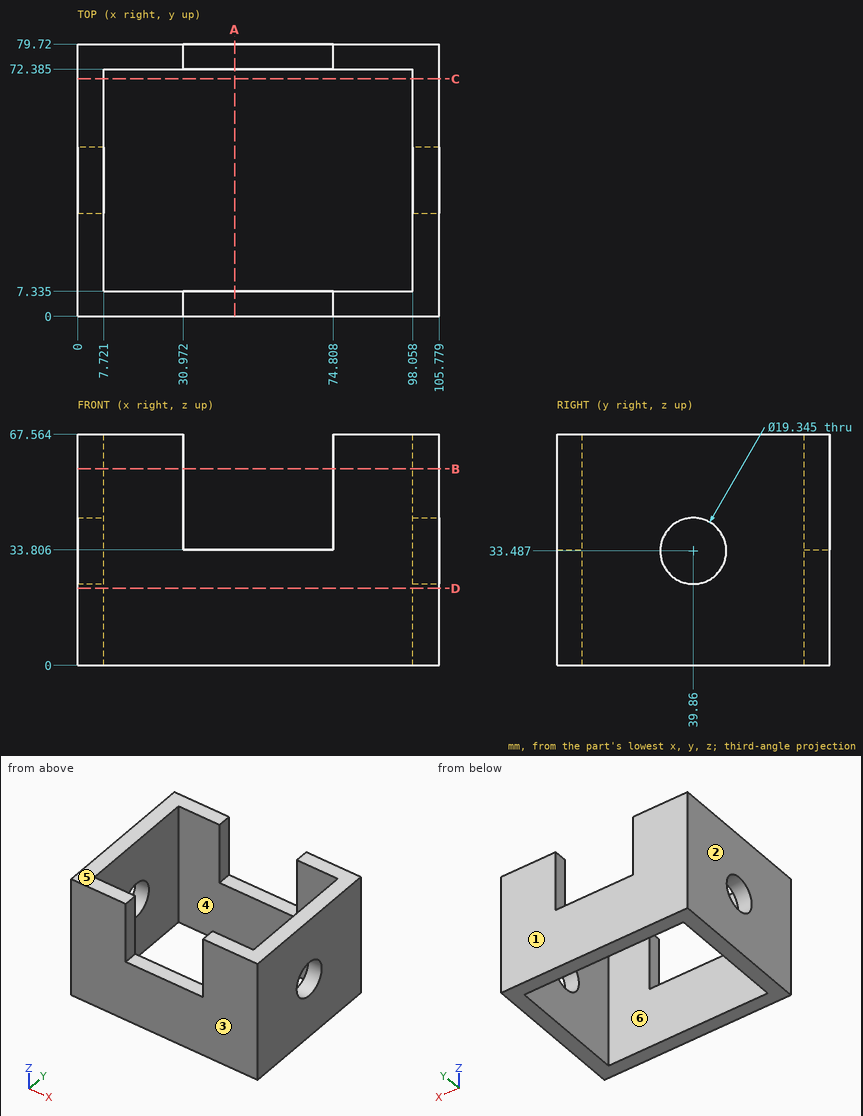
The figure shows three views and two pictorial views of one solid part (mm, origin at its lowest corner). Answer the questions. A direction names the side the tool comes from. Give positions to 0.01 mm unless a question says otherwise; leave off trailing zeros. Write each loop counter-clockwise with the first axis right and the second up, starting at its lowest first coordinate (ties: lowest second). Pieces come first, ordered by that corner, then holes. Notation, with made-up numbers: M -34.5,87.25 L 2.5,87.25 A15 cw 2.5,100.25 Z; hole C 23.5,62.5 d7. An arc over 180 degrees is marked long. One line per item, written item: value. Start each with the question number.
(1) A flat-ended cylindrical pin translates along its axis: pin 1 Ø6 at (x, y) = (47, 3.5) entering from +Z. Find the tip coordinate at first contact, or state that the pin passes through.
(2) Determine the mould class of the marked faces 1, 2, 3 and 4 for opening direction Y: pulls with the +Y half, pulls with the -Y half, needs draft (parallel to the pull), parting line crosses it, or undercut.
(3) Find the intervals of material crossed by line 1 (X direction, y = 30.5, z = 60.5); line 2 (Y direction, x = 94.5, z = 30) (1 decimal); line 3 (Z direction, x = 66.5, y = 73.5) (1 decimal), in increasing order.
(4) Find section B-B (z = 57.5). Determine the outline of the cut face in (x, y) (1 decimal).
(5) A tool of negligible diameter and unlimited length cuts with its end or side. For the marked faces 5 and 6, from which of +Z, -Z, +X, -X, +Y, -Y can it reach the whole face along a straight path? Write none if from no direction.
(6) Find section D-D (z = 22.5). Determine the outline of the cut face in (x, y) (1 decimal).
(7) Find section A-A (x = 46). Determine the outline of the cut face in (y, z) (1 decimal), plus the area to 3 significant figures.
(8) Find section C-C (y = 69.5). Determine the outline of the cut face in (x, z) (1 decimal), plus the area to 3 significant figures.
Results below:
1. pin 1: stops at z = 33.81
2. face 1: pulls with the +Y half
2. face 2: needs draft
2. face 3: pulls with the -Y half
2. face 4: undercut
3. line 1: x = 0 to 7.72, 98.06 to 105.78
3. line 2: y = 0 to 7.3, 72.4 to 79.7
3. line 3: z = 0 to 33.8
4. outline: M 0,0 L 31,0 L 31,7.3 L 7.7,7.3 L 7.7,72.4 L 31,72.4 L 31,79.7 L 0,79.7 Z; M 74.8,0 L 105.8,0 L 105.8,79.7 L 74.8,79.7 L 74.8,72.4 L 98.1,72.4 L 98.1,7.3 L 74.8,7.3 Z
5. face 5: +Z, +X, -X, +Y, -Y
5. face 6: +Z, -Z
6. outline: M 0,0 L 105.8,0 L 105.8,79.7 L 0,79.7 Z; hole M 7.7,7.3 L 98.1,7.3 L 98.1,72.4 L 7.7,72.4 Z
7. outline: M 0,0 L 7.3,0 L 7.3,33.8 L 0,33.8 Z; M 72.4,0 L 79.7,0 L 79.7,33.8 L 72.4,33.8 Z
7. area: 496 mm^2
8. outline: M 0,0 L 7.7,0 L 7.7,67.6 L 0,67.6 Z; M 98.1,0 L 105.8,0 L 105.8,67.6 L 98.1,67.6 Z
8. area: 1,040 mm^2
